Source: CAD feature listing. Evaluate the final solid. Frame: model axes, mm. A direction names the side the tool comes from. Round coordinates to 2 decimals unless told otherwise and drop trailing zeros. Write each loop counter-clockwise with the first axis right and the second up, starting at its lowest first coordinate (ties: lowest second). Pieces come first, ordered by that corner, then holes. Notation, with made-up numbers: M 67,60.25 L 125,60.25 A9 cw 125,76.25 Z; hole C 15.5,-33 d1. An arc over 180 degrees is marked long. Answer in a Markdown table with one row per item. Add a question column.
Item 1: Mould query, pull axis Y, two halves, no side actions, for faces 1 (the face through (30, 37.328, 8)), 2 (the face through (41, 49, 8)), 3 (the face through (40, 25, 10)). Classes: released by +Y, released by -Y, zero draft, split by the parting line, or undercut.
Item 2: Cut plane D-D on x = 53.5. Return loops of the section in (y, z).
Item 3: Cut plane A-A on y = 13.5. Return loops of the section in (x, z), and give its area (3 significant figures).
Item 4: Set-up query: faces 4 (the face through (80, 25, 2)), 5 (the face through (55.5, 13, 8)). Return all of +Z, -Z, +X, -X, +Y, -Y with unobstructed straight access to the full face (end or side cutting, diameter ignored); none if empty.
Item 5: Contact query for flat-ended pins moving along their axis: pin 1 (1.5 mm diameter, centred on x = 63.5, z = 7, fed in from +Y); pin 2 (3 mm diameter, centred on y = 37.5, z = 9, fed in from -X); pin 3 (5.5 mm diameter, centred on x = 48.5, z = 8, fed in from +Y). Output: stop coordinate, or through.
Item 6: Material intervals for probe 1 along X at (y, z) = (29, 5.25); probe 2 along X at (y, z) = (21.5, 5.75); probe 3 along Z at (x, y) = (59.5, 14), sorted ascending.
Item 7: Cut plane C-C on x = 29. Return loops of the section in (y, z).
Item 8: Cut plane B-B on z = 7.75. Give the number of separate pieces and of enclosed holes in the cut face, and give its area (3 significant figures).
from build123d import *

# Parameters (mm, degrees)
F0_W     = 80
F0_H     = 50
F1_DEPTH = 10
F2_W     = 5
F2_H     = 25
F2_H_2   = 26.404956
F3_DEPTH = 5
F4_R     = 5


with BuildPart() as f1:
    # F0 (on Top) → F1 (new body)
    with BuildSketch(Plane.XY):
        with Locations((40, 25)):
            Rectangle(F0_W, F0_H)
    extrude(amount=F1_DEPTH)

    # F2 (on face) → F3 (cut)
    with BuildSketch(Plane.XY.offset(10)):
        with Locations((12, 24.827586)):
            Rectangle(F2_W, F2_H)
        Polygon((26.5, 30.92263), (26.5, 10.92263), (33.5, 10.92263), (33.5, 30.92263), (40.5, 30.92263), (40.5, 37.327586), (19.5, 37.327586), (19.5, 30.92263), align=None)
        with Locations((48, 24.125108)):
            Rectangle(F2_W, F2_H_2)
        Polygon((70.5, 32.327586), (70.5, 37.327586), (55.5, 37.327586), (55.5, 21.92263), (64.5, 21.92263), (64.5, 15.92263), (55.5, 15.92263), (55.5, 10.92263), (70.5, 10.92263), (70.5, 26.327586), (60.5, 26.327586), (60.5, 32.327586), align=None)
    extrude(amount=-F3_DEPTH, mode=Mode.SUBTRACT)

    # F4
    f4_edges = [f1.edges().sort_by_distance(p)[0] for p in [
        (0, 25, 10),
        (40, 0, 10),
        (80, 25, 10),
        (40, 50, 10),
    ]]
    fillet(f4_edges, radius=F4_R)


solid = f1.part
Results below:
| question | item | result |
|---|---|---|
| 1 | face 1 | undercut |
| 1 | face 2 | released by +Y |
| 1 | face 3 | zero draft |
| 2 | outline | M 0,0 L 50,0 L 50,5 A5 ccw 45,10 L 5,10 A5 ccw 0,5 Z |
| 3 | outline | M 0,0 L 80,0 L 80,5 A5 ccw 75,10 L 70.5,10 L 70.5,5 L 55.5,5 L 55.5,10 L 50.5,10 L 50.5,5 L 45.5,5 L 45.5,10 L 33.5,10 L 33.5,5 L 26.5,5 L 26.5,10 L 14.5,10 L 14.5,5 L 9.5,5 L 9.5,10 L 5,10 A5 ccw 0,5 Z |
| 3 | area | 629 mm2 |
| 4 | face 4 | +Z, -Z, +X, +Y, -Y |
| 4 | face 5 | +Z |
| 5 | pin 1 | y = 49.84 |
| 5 | pin 2 | x = 0.67 |
| 5 | pin 3 | y = 49.99 |
| 6 | probe 1 | 0.01 to 9.5, 14.5 to 26.5, 33.5 to 45.5, 50.5 to 55.5, 60.5 to 79.99 |
| 6 | probe 2 | 0.06 to 9.5, 14.5 to 26.5, 33.5 to 45.5, 50.5 to 64.5, 70.5 to 79.94 |
| 6 | probe 3 | 0 to 5 |
| 7 | outline | M 0,0 L 50,0 L 50,5 A5 ccw 45,10 L 37.33,10 L 37.33,5 L 10.92,5 L 10.92,10 L 5,10 A5 ccw 0,5 Z |
| 8 | separate pieces | 1 |
| 8 | enclosed holes | 4 |
| 8 | area | 2,970 mm2 |
